```python
from build123d import *

# Parameters (mm, degrees)
SKETCH1_W           = 40
SKETCH1_H           = 40
BOSS_EXTRUDE1_DEPTH = 40
SKETCH2_R           = 7.5
BOSS_EXTRUDE2_DEPTH = 17.5
SKETCH3_R           = 7.5
BOSS_EXTRUDE3_DEPTH = 17.5


with BuildPart() as part:
    # Sketch1 → Boss-Extrude1 (new body)
    with BuildSketch(Plane.XY):
        Rectangle(SKETCH1_W, SKETCH1_H)
    extrude(amount=BOSS_EXTRUDE1_DEPTH)

    # Sketch2 → Boss-Extrude2 (add)
    with BuildSketch(Plane(origin=(0, 20, 0), x_dir=(1, 0, 0), z_dir=(0, 1, 0))):
        with Locations(Location((0, -20, 0), (0, 0, 270))):
            Circle(SKETCH2_R)
    boss_extrude2 = extrude(amount=BOSS_EXTRUDE2_DEPTH)

    # Mirror1: Boss-Extrude2 across plane
    add(boss_extrude2.mirror(Plane.ZX))

    # Sketch3 → Boss-Extrude3 (add)
    with BuildSketch(Plane(origin=(20, 0, 0), x_dir=(0, 0, -1), z_dir=(1, 0, 0))):
        with Locations((-20, 0)):
            Circle(SKETCH3_R)
    boss_extrude3 = extrude(amount=BOSS_EXTRUDE3_DEPTH)

    # Mirror2: Boss-Extrude3 across plane
    add(boss_extrude3.mirror(Plane(origin=(0, 0, 0), x_dir=(0, 0, 1), z_dir=(1, 0, 0))))


solid = part.part
```
For this review, take the finished solid that the model builds, in its own axes (mm). A direction names the side the tool comes from. Round coordinates to 2 decimals unless told otherwise and drop trailing zeros. Loops run counter-clockwise (first coordinate to the right, second up) from the corner with the lowest first, then second, coordinate; pieces in that order, holes last.
Q1. Add section C-C on y = 0. Write out the cut boundary in (x, z).
Result sheet:
outline: (-37.5, 12.5) - (-20, 12.5) - (-20, 0) - (20, 0) - (20, 12.5) - (37.5, 12.5) - (37.5, 27.5) - (20, 27.5) - (20, 40) - (-20, 40) - (-20, 27.5) - (-37.5, 27.5) - close
Q2. Add section B-B on x = -6. Write out the cut boundary in (y, z).
Result sheet:
outline: (-37.5, 15.5) - (-20, 15.5) - (-20, 0) - (20, 0) - (20, 15.5) - (37.5, 15.5) - (37.5, 24.5) - (20, 24.5) - (20, 40) - (-20, 40) - (-20, 24.5) - (-37.5, 24.5) - close
Q3. Machinability: for faces 1 (the face through (-20, 0, 11)), 2 (the face through (0.33, 28.627, 12.507)), 3 (the face through (0, 0, 0)), 4 (the face through (20, 0, 11)), 5 (the face through (0.33, -28.627, 12.507)), which of the approach directions +Z, -Z, +X, -X, +Y, -Y give a long, thin tool a straight path to every point of the face, cutting with its end or side? Answer none if there is none.
Result sheet:
face 1: -X
face 2: +Y
face 3: -Z, +X, -X, +Y, -Y
face 4: +X
face 5: -Y
Q4. Insertion check: pin 1 Ø2 at (x, z) = (12, 29) entering from -Y; pin 2 Ø1.5 at (y, z) = (-22, 23.5) entering from +X; pin 3 Ø6 at (x, z) = (-18, 25.5) entering from +Y. Each pin has a flat end and moves straight along its axis. Give the tip position at first contact, or say it passes through.
Result sheet:
pin 1: stops at y = -20
pin 2: stops at x = 6.98
pin 3: stops at y = 20
Q5. Add section A-A on z = 26. Write out the cut boundary in (x, y).
Result sheet:
outline: (-37.5, -4.5) - (-20, -4.5) - (-20, -20) - (-4.5, -20) - (-4.5, -37.5) - (4.5, -37.5) - (4.5, -20) - (20, -20) - (20, -4.5) - (37.5, -4.5) - (37.5, 4.5) - (20, 4.5) - (20, 20) - (4.5, 20) - (4.5, 37.5) - (-4.5, 37.5) - (-4.5, 20) - (-20, 20) - (-20, 4.5) - (-37.5, 4.5) - close
Q6. To check wall thickness, follow line 1 along X through (y, z) = (-13.5, 3); line 2 along Y through (x, z) = (-21, 22). State the ranges of each line that lie inside material, in increasing order.
Result sheet:
line 1: x = -20 to 20
line 2: y = -7.23 to 7.23
Q7. Add section D-D on z = 20. Write out the cut boundary in (x, y), plus the area to 3 significant figures.
Result sheet:
outline: (-37.5, -7.5) - (-20, -7.5) - (-20, -20) - (-7.5, -20) - (-7.5, -37.5) - (7.5, -37.5) - (7.5, -20) - (20, -20) - (20, -7.5) - (37.5, -7.5) - (37.5, 7.5) - (20, 7.5) - (20, 20) - (7.5, 20) - (7.5, 37.5) - (-7.5, 37.5) - (-7.5, 20) - (-20, 20) - (-20, 7.5) - (-37.5, 7.5) - close
area: 2,650 mm2
